Source: CAD feature listing. Evaluate the final solid. Frame: model axes, mm. A direction names the side the tool comes from. Give positions to 0.01 mm unless a question says otherwise; leave off trailing zeros. Write each loop counter-clockwise with the first axis right and the second up, starting at its lowest first coordinate (ties: lowest second). Pieces come first, ordered by that corner, then holes. Notation, with made-up numbers: M -40,-26 L -6,-26 A17 ccw -6,6 Z; hole C 88.25,61 d10. An arc over 180 degrees is marked long. Answer as a JSON object with one key per item and string values. Group by question number.
```python
from build123d import *

# Parameters (mm, degrees)
BOSS_EXTRU_1_DEPTH      = 5
ESQUISSE3_R             = 16.5
BOSS_EXTRU_2_DEPTH      = 15
ESQUISSE4_R             = 16.5
BOSS_EXTRU_3_DEPTH      = 5
ESQUISSE5_R             = 5
ENL_V_MAT_EXTRU_1_DEPTH = 26
ESQUISSE6_R             = 4.5
ENL_V_MAT_EXTRU_2_DEPTH = 5
CONG_1_R                = 0.5
CHANFREIN1_SIZE         = 0.5


with BuildPart() as part:
    # Esquisse2 → Boss.-Extru.1 (new body)
    with BuildSketch(Plane.XY):
        with BuildLine():
            Line((-37.5, 4.330127019), (-2.5, 24.537386441))
            ThreePointArc((-2.5, 24.537386441), (0, 25.207259422), (2.5, 24.537386441))
            Line((2.5, 24.537386441), (37.5, 4.330127019))
            ThreePointArc((37.5, 4.330127019), (40, 0), (37.5, -4.330127019))
            Line((37.5, -4.330127019), (2.5, -24.537386441))
            ThreePointArc((2.5, -24.537386441), (0, -25.207259422), (-2.5, -24.537386441))
            Line((-2.5, -24.537386441), (-37.5, -4.330127019))
            ThreePointArc((-37.5, -4.330127019), (-40, 0), (-37.5, 4.330127019))
        make_face()
    extrude(amount=BOSS_EXTRU_1_DEPTH)

    # Esquisse3 → Boss.-Extru.2 (add)
    with BuildSketch(Plane.XY.offset(5)):
        with Locations(Location((0, 0, 0), (0, 0, 180))):  # turned: the seam where the file's is
            Circle(ESQUISSE3_R)
    extrude(amount=BOSS_EXTRU_2_DEPTH)

    # Esquisse4 → Boss.-Extru.3 (add)
    with BuildSketch(Plane(origin=(0, 0, 0), x_dir=(-1, 0, 0), z_dir=(0, 0, -1))):
        Circle(ESQUISSE4_R)
    extrude(amount=BOSS_EXTRU_3_DEPTH)

    # Esquisse5 → Enlèv. mat.-Extru.1 (cut, through all)
    with BuildSketch(Plane(origin=(0, 0, -5), x_dir=(-1, 0, 0), z_dir=(0, 0, -1))):
        Circle(ESQUISSE5_R)
    extrude(amount=-ENL_V_MAT_EXTRU_1_DEPTH, mode=Mode.SUBTRACT)

    # Esquisse6 → Enlèv. mat.-Extru.2 (cut)
    with BuildSketch(Plane.XY.offset(5)):
        with Locations((29.5, 0)):
            Circle(ESQUISSE6_R)
        with Locations((-29.5, 0)):
            Circle(ESQUISSE6_R)
    extrude(amount=-ENL_V_MAT_EXTRU_2_DEPTH, mode=Mode.SUBTRACT)

    # Congé1
    cong_1_edges = [part.edges().sort_by_distance(p)[0] for p in [
        (16.5, 0, 5),
        (16.5, 0, 0),
    ]]
    fillet(cong_1_edges, radius=CONG_1_R)

    # Chanfrein1
    chanfrein1_edges = [part.edges().sort_by_distance(p)[0] for p in [
        (16.5, 0, 20),
    ]]
    chamfer(chanfrein1_edges, length=CHANFREIN1_SIZE)


solid = part.part
```
(1) Pull-direction query (Y, two-part tool) for faces 4 (the flat face through (-20.245, 14.292, 2.465)), 5 (the cylindrical face through (-15.738, -4.956, 12.402)), 6 (the cylindrical face through (-25.208, 1.352, 2.535)), 7 (the cylindrical face through (33.792, 1.352, 2.535)); classes: pulls with the +Y half, pulls with the -Y half, needs draft (parallel to the pull), parting line crosses it, or undercut.
(2) Section B-B, the plane x = 0. Return loops of the section in (y, z), plus the area to 3 significant figures.
(3) Section A-A, the plane y = 0. State how many separate pieces and enclosed holes the cut face has, plus the area to 3 significant figures.
(4) Contact query for flat-ended pins moving along their axis: pin 1 Ø6 at (x, y) = (-24, 8) entering from +Z; pin 2 Ø3 at (x, z) = (-26.5, 4.5) entering from +Y; pin 3 Ø5 at (y, z) = (-6, 17) entering from +X. Output: stop coordinate, or through.
(5) Ray query, L1, parallel to Y at x = 0, z = 15; L2, parallel to Y at x = 0, z = 3.75; L3, parallel to Z at x = 20, y = -3.5. Return the intervals inside material, ascending. Write a range as [from, to].
(6) Section C-C, the plane z = 11.25. Return loops of the section in (x, y), plus the area to 3 significant figures.
(7) Access query for faces 1 (the cylindrical face through (1.08, -4.88, 7.32)), 2 (the flat face through (-9, -15, 0)), 3 (the flat face through (-9, -15, 5)). Directions: +Z, -Z, +X, -X, +Y, -Y. A direction counts if a zero-diameter tool reaches every point of the face in a straight line with its end or side. Return the directions, or none.
(8) Section D-D, the plane x = 29.5. Return loops of the section in (y, z).
Reported:
{
 "1": {"face 4": "pulls with the +Y half", "face 5": "parting line crosses it", "face 6": "undercut", "face 7": "undercut"},
 "2": {"outline": "M -25.21,0 L -17,0 A0.5 cw -16.5,-0.5 L -16.5,-5 L -5,-5 L -5,20 L -16,20 L -16.5,19.5 L -16.5,5.5 A0.5 cw -17,5 L -25.21,5 Z; M 5,-5 L 16.5,-5 L 16.5,-0.5 A0.5 cw 17,0 L 25.21,0 L 25.21,5 L 17,5 A0.5 cw 16.5,5.5 L 16.5,19.5 L 16,20 L 5,20 Z", "area": "662 mm2"},
 "3": {"separate pieces": "4", "enclosed holes": "0", "area": "720 mm2"},
 "4": {"pin 1": "stops at z = 5", "pin 2": "stops at y = 11.55", "pin 3": "stops at x = 16.12"},
 "5": {"L1": "y = [-16.5, -5], [5, 16.5]", "L2": "y = [-25.21, -5], [5, 25.21]", "L3": "z = [0, 5]"},
 "6": {"outline": "C 0,0 d33; hole C 0,0 d10", "area": "777 mm2"},
 "7": {"face 1": "+Z, -Z", "face 2": "-Z", "face 3": "+Z"},
 "8": {"outline": "M -8.95,0 L -4.5,0 L -4.5,5 L -8.95,5 Z; M 4.5,0 L 8.95,0 L 8.95,5 L 4.5,5 Z"}
}
